CAD build for the part. Positions are in the model's coordinates, mm. Round coordinates to 2 decimals unless told otherwise and drop trailing zeros. Write each loop counter-clockwise with the first axis right and the second up, starting at its lowest first coordinate (ties: lowest second). Pieces come first, ordered by that corner, then holes. Notation, with made-up numbers: (-38.75, -22) -> (-1.75, -22) arc R16 ccw to (-1.75, 0) -> close; hole circle Ø3 at (84.5, 16.5). An arc over 180 degrees is marked (long way). Answer in a Markdown table with one row per item. Add a question column.
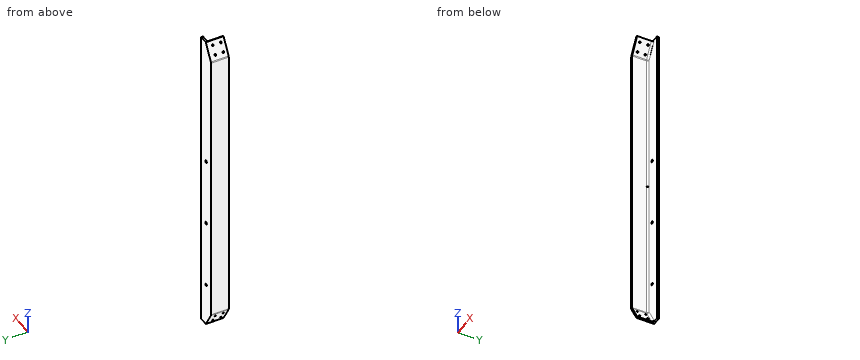
```python
from build123d import *

# Parameters (mm, degrees)
BOSS_EXTRUDE1_DEPTH  = 640
BOSS_EXTRUDE2_DEPTH  = 8
BOSS_EXTRUDE3_DEPTH  = 72
SKETCH6_R            = 4
CUT_EXTRUDE1_DEPTH   = 8
FILLET1_R            = 10
FILLET2_R            = 8
FILLET1_OF_MIRROR1_R = 10
FILLET2_OF_MIRROR1_R = 8
SKETCH10_R           = 6
CUT_EXTRUDE2_DEPTH   = 8


with BuildPart() as part:
    # Sketch1 → Boss-Extrude1 (new body)
    with BuildSketch(Plane.XY):
        Polygon((-8, 8), (72, 8), (72, 0), (0, 0), (0, -72), (-8, -72), align=None)
    boss_extrude1 = extrude(amount=BOSS_EXTRUDE1_DEPTH)

    # Sketch3 → Boss-Extrude2 (add)
    with BuildSketch(Plane(origin=(0, 0, 0), x_dir=(1, 0, 0), z_dir=(0, 1, 0))):
        Polygon((-8, -640), (34.5, -713.612159322), (72, -713.612159322), (72, -640), align=None)
    boss_extrude2 = extrude(amount=BOSS_EXTRUDE2_DEPTH)

    # Sketch4 → Boss-Extrude3 (add)
    with BuildSketch(Plane.XZ):
        Polygon((-8, 640), (34.5, 713.612159322), (40.5, 710.148057707), (0, 640), align=None)
    boss_extrude3 = extrude(amount=BOSS_EXTRUDE3_DEPTH)

    # Sketch6 → Cut-Extrude1 (cut)
    with BuildSketch(Plane(origin=(-277.128129211, 0, 160), x_dir=(-0.4999999999999956, 0, -0.8660254037844413), z_dir=(0.8660254037844413, 0, -0.4999999999999956))):
        with Locations((-615.006258422, -18)):
            Circle(SKETCH6_R)
        with Locations((-574.506258422, -18)):
            Circle(SKETCH6_R)
        with Locations((-574.506258422, -54)):
            Circle(SKETCH6_R)
        with Locations((-615.006258422, -54)):
            Circle(SKETCH6_R)
    cut_extrude1 = extrude(amount=-CUT_EXTRUDE1_DEPTH, mode=Mode.SUBTRACT)

    # Fillet1
    fillet1_edges = [part.edges().sort_by_distance(p)[0] for p in [
        (0, -36, 640),
        (-8, -32, 640),
    ]]
    fillet(fillet1_edges, radius=FILLET1_R)

    # Fillet2
    fillet2_edges = [part.edges().sort_by_distance(p)[0] for p in [
        (20.919872981, 0, 676.234282891),
        (0, 0, 318.660254038),
        (0.340741737, 0, 639.908698527),
    ]]
    fillet(fillet2_edges, radius=FILLET2_R)

    # Mirror1: Boss-Extrude1, Boss-Extrude2, Boss-Extrude3, Cut-Extrude1 across plane
    add(boss_extrude1.mirror(Plane.XY))
    add(boss_extrude2.mirror(Plane.XY))
    add(boss_extrude3.mirror(Plane.XY))
    add(cut_extrude1.mirror(Plane.XY), mode=Mode.SUBTRACT)

    # Fillet1 of Mirror1
    fillet1_of_mirror1_edges = [part.edges().sort_by_distance(p)[0] for p in [
        (0, -36, -640),
        (-8, -32, -640),
    ]]
    fillet(fillet1_of_mirror1_edges, radius=FILLET1_OF_MIRROR1_R)

    # Fillet2 of Mirror1
    fillet2_of_mirror1_edges = [part.edges().sort_by_distance(p)[0] for p in [
        (20.919872981, 0, -676.234282891),
        (0, 0, -318.660254038),
        (0.340741737, 0, -639.908698527),
    ]]
    fillet(fillet2_of_mirror1_edges, radius=FILLET2_OF_MIRROR1_R)

    # Sketch10 → Cut-Extrude2 (cut)
    with BuildSketch(Plane(origin=(0, 8, 0), x_dir=(1, 0, 0), z_dir=(0, 1, 0))):
        with Locations(Location((32, 513.612159322, 0), (0, 0, 180))):
            Circle(SKETCH10_R)
        with Locations(Location((32, 201.112159322, 0), (0, 0, 180))):
            Circle(SKETCH10_R)
        with Locations(Location((32, -110.512159322, 0), (0, 0, 180))):
            Circle(SKETCH10_R)
    extrude(amount=-CUT_EXTRUDE2_DEPTH, mode=Mode.SUBTRACT)


solid = part.part
```
Item 1: Pin check, flat tips, straight feed: pin 1 (14 mm diameter, centred on x = 32, z = -201.11, fed in from +Y); pin 2 (2 mm diameter, centred on x = 57.5, z = -63.5, fed in from -Y); pin 3 (9 mm diameter, centred on x = 5.5, y = -5.5, fed in from -Z); pin 4 (4 mm diameter, centred on x = 3.5, y = -5, fed in from +Z). Stop position of each tip, or through.
Item 2: Saw through at A-A on z = 517.5. Give the cut face in (x, y), then the cut area to 3 significant figures.
Item 3: Saw through at B-B on x = 59. Give the cut face in (y, z), then the cut area to 3 significant figures.
Item 4: Drill centre lines: probe 1 along Z at (x, y) = (32, 3.75); probe 2 along X at (y, z) = (-24, 160.5); probe 3 along Y at (x, z) = (50, -450.5). Where is each one in solid material? Low to high.
Recorded:
| question | item | result |
|---|---|---|
| 1 | pin 1 | y = 8 |
| 1 | pin 2 | y = 0 |
| 1 | pin 3 | z = -671.18 |
| 1 | pin 4 | z = 663.38 |
| 2 | outline | (-8, -72) -> (0, -72) -> (0, -8) arc R8 cw to (8, 0) -> (72, 0) -> (72, 8) -> (-8, 8) -> close |
| 2 | area | 1,230 mm2 |
| 3 | outline | (0, -713.61) -> (8, -713.61) -> (8, 713.61) -> (0, 713.61) -> close |
| 3 | area | 11,400 mm2 |
| 4 | probe 1 | -709.28 to -519.61, -507.61 to -207.11, -195.11 to 104.51, 116.51 to 709.28 |
| 4 | probe 2 | -8 to 0 |
| 4 | probe 3 | 0 to 8 |
